Check sheet for the modelled part. Datum: model origin and axes. Units: mm. Round coordinates to 2 decimals unless told otherwise and drop trailing zeros. Order: outer loops, then holes, each group sorted by start corner. A loop starts at its lowest first (then second) coordinate and runs counter-clockwise, first axis right, second up.
(1) Sectioned sample at C-C, the plane x = 18. Enter the section's corners in (y, z), and give its area (3 significant figures).
(2) Sectioned sample at B-B, the plane y = 0.75. Enter the section's corners in (x, z), and give its area (3 significant figures).
(3) Depth check by flat-ended pin: pin 1 (4 mm diameter, centred on x = 28, y = -2.5, fed in from +Z). Enter the tip coordinate at first touch or a pass-through.
(4) Sectioned sample at D-D, the plane z = 129. Enter the section's corners in (x, y).
(5) Thickness scan on probe 1 along Z at (x, y) = (37, -2); probe 2 along X at (y, z) = (-1.75, -69.5); probe 3 along Z at (x, y) = (38, -1.25). Record the ranges inside material, lowest first.
(6) Sectioned sample at A-A, the plane z = -37.5. Enter the section's corners in (x, y), and give its area (3 significant figures).
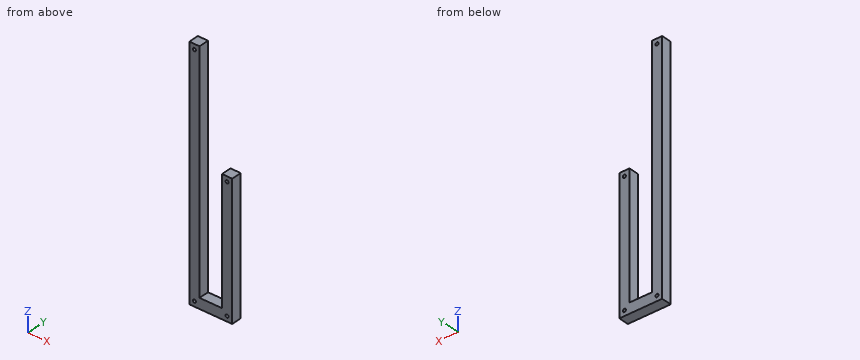
```python
from build123d import *

# Parameters (mm, degrees)
F0_R     = 1.5
F0_W     = 22
F0_H     = 10
F1_DEPTH = 5
F2_DEPTH = 5


# Not quite as in the source:
# - a feature names something its author has since deleted; it is built from what else it names


with BuildPart() as f1:
    # F0 (on Front) → F1 (new body, symmetric)
    with BuildSketch(Plane.XZ):
        Polygon((10, 147.8899265081), (0, 147.8899265081), (0, -87.1100734919), (10, -87.1100734919), (10, -77.1100734919), align=None)
        with Locations((5, -82.1100734919)):
            Circle(F0_R, mode=Mode.SUBTRACT)
        with Locations((5, 142.8899265081)):
            Circle(F0_R, mode=Mode.SUBTRACT)
        with Locations((21, -82.1100734919)):
            Rectangle(F0_W, F0_H)
        Polygon((32, 42.8899265081), (32, -77.1100734919), (32, -87.1100734919), (42, -87.1100734919), (42, 42.8899265081), align=None)
        with Locations((37, -82.1100734919)):
            Circle(F0_R, mode=Mode.SUBTRACT)
        with Locations((37, 37.8899265081)):
            Circle(F0_R, mode=Mode.SUBTRACT)
    extrude(amount=F1_DEPTH, both=True)

    # F0 (on Front) → F2 (cut, symmetric)
    with BuildSketch(Plane.XZ):
        with Locations((5, -82.1100734919)):
            Circle(F0_R)
        with Locations((37, -82.1100734919)):
            Circle(F0_R)
        with Locations((37, 37.8899265081)):
            Circle(F0_R)
        with Locations((5, 142.8899265081)):
            Circle(F0_R)
    extrude(amount=F2_DEPTH, both=True, mode=Mode.SUBTRACT)


solid = f1.part
```
Derived:
1. outline: (-5, -87.11) - (5, -87.11) - (5, -77.11) - (-5, -77.11) - close
1. area: 100 mm2
2. outline: (0, -87.11) - (42, -87.11) - (42, 42.89) - (32, 42.89) - (32, -77.11) - (10, -77.11) - (10, 147.89) - (0, 147.89) - close; hole circle Ø3 at (5, -82.11); hole circle Ø3 at (5, 142.89); hole circle Ø3 at (37, -82.11); hole circle Ø3 at (37, 37.89)
2. area: 3,840 mm2
3. pin 1: stops at z = -77.11
4. outline: (0, -5) - (10, -5) - (10, 5) - (0, 5) - close
5. probe 1: z = -87.11 to -83.61, -80.61 to 36.39, 39.39 to 42.89
5. probe 2: x = 0 to 10, 32 to 42
5. probe 3: z = -87.11 to -83.23, -80.99 to 36.77, 39.01 to 42.89
6. outline: (0, -5) - (10, -5) - (10, 5) - (0, 5) - close; (32, -5) - (42, -5) - (42, 5) - (32, 5) - close
6. area: 200 mm2
